```python
from build123d import *

# Parameters (mm, degrees)
F1_ANGLE = 183.776526


with BuildPart() as f1:
    # F0 (on Front) → F1 (revolve, symmetric)
    with BuildSketch(Plane.XZ) as f1_sk:
        with BuildLine():
            ThreePointArc((15, 38.610307), (-0.039705, 41.242922), (-15, 38.191206))
            Line((-15, 38.191206), (-14.952645, 35.732973))
            Line((-14.952645, 35.732973), (-15, 35.708816))
            Line((-15, 35.708816), (-15, 34.639609))
            Line((-15, 34.639609), (-14.340117, 34.990203))
            Line((-14.340117, 34.990203), (-14.340117, 36.578923))
            ThreePointArc((-14.340117, 36.578923), (-0.01537, 39.500995), (14.385413, 36.98022))
            Line((14.385413, 36.98022), (14.385413, 35.022542))
            Line((14.385413, 35.022542), (15, 34.765044))
            Line((15, 34.765044), (15, 35.966083))
            Line((15, 35.966083), (15, 38.610307))
        make_face()
    revolve(axis=Axis((0.706701, 0, 7.158781), (0.999932, 0, 0.011679)), revolution_arc=F1_ANGLE / 2)
    revolve(f1_sk.sketch, axis=Axis((0.706701, 0, 7.158781), (-0.999932, 0, -0.011679)), revolution_arc=F1_ANGLE / 2)


solid = f1.part
```
Can you work these out from the model? Positions are in its coordinate system, mm. Coordinates: 2 decimals unless noted, no trailing zeros. Put each result on its own line as item: value. Start each with the question number.
(1) We'd pull the mould along Y, two halves only. Please class faces 1 (the face through (14.83, -0.62, 34.83)), 2 (the face through (14.385, -0.629, 35.328)): +Y half, -Y half, draft (parallel to the pull), parting line (faces both ways), or undercut.
(2) I need wall thicknesses on probe 1 along Y at (x, z) = (9.5, 20); probe 2 along Y at (x, z) = (10, 13); probe 3 along Z at (x, y) = (-10.5, -16). Which ranges of each line are inside material? Lowest first, please.
(3) Will these pins go through, and if not, where does the flat tip stop? pin 1 Ø2 at (x, z) = (-8.5, 34) entering from +Y; pin 2 Ø1.5 at (x, z) = (4, 21) entering from +Y; pin 3 Ø4 at (x, z) = (1, 9.5) entering from -Y; pin 4 Ø6 at (y, z) = (-13, 26) entering from +X.
Worked answers:
1. face 1: undercut
1. face 2: undercut
2. probe 1: y = -30.49 to -28.54, 28.54 to 30.49
2. probe 2: y = -32.44 to -30.62, 30.62 to 32.44
2. probe 3: z = 33.44 to 35.54
3. pin 1: stops at y = 20.71
3. pin 2: stops at y = 31.32
3. pin 3: stops at y = -34.09
3. pin 4: passes through
